```python
from build123d import *

# Parameters (mm, degrees)
BOSS_EXTRUDE1_DEPTH = 12.7
CUT_EXTRUDE1_START  = -13.7
SKETCH2_R           = 2.5
CUT_EXTRUDE1_DEPTH  = 14.7
LPATTERN1_COUNT     = 11
LPATTERN1_PITCH     = 38.608
CUT_EXTRUDE2_START  = -13.7
SKETCH3_R           = 2.5
CUT_EXTRUDE2_DEPTH  = 14.7
LPATTERN2_COUNT     = 11
LPATTERN2_PITCH     = 38.608
CUT_EXTRUDE3_START  = -13.7
SKETCH4_R           = 2.5
CUT_EXTRUDE3_DEPTH  = 14.7
LPATTERN3_COUNT     = 12
LPATTERN3_PITCH     = 38.608
CUT_EXTRUDE4_START  = -13.7
SKETCH5_R           = 2.5
CUT_EXTRUDE4_DEPTH  = 14.7
LPATTERN4_COUNT     = 12
LPATTERN4_PITCH     = 38.608


with BuildPart() as part:
    # Sketch1 → Boss-Extrude1 (new body)
    with BuildSketch(Plane(origin=(0, 0, 0), x_dir=(1, 0, 0), z_dir=(0, 1, 0))):
        Polygon((-199.53099264, 245.600086338), (200.46900736, 245.600086338), (200.46900736, 225.600086338), (240.46900736, 225.600086338), (240.46900736, -224.399913662), (200.46900736, -224.399913662), (200.46900736, -244.399913662), (-199.53099264, -244.399913662), (-199.53099264, -224.399913662), (-239.53099264, -224.399913662), (-239.53099264, 225.600086338), (-199.53099264, 225.600086338), align=None)
    extrude(amount=BOSS_EXTRUDE1_DEPTH)

    # Sketch2 → Cut-Extrude1 (cut)
    with BuildSketch(Plane(origin=(0, 12.7, 0), x_dir=(1, 0, 0), z_dir=(0, 1, 0)).offset(CUT_EXTRUDE1_START)):
        with Locations((-192.67299264, 235.440086338)):
            Circle(SKETCH2_R)
    cut_extrude1 = extrude(amount=CUT_EXTRUDE1_DEPTH, mode=Mode.SUBTRACT)

    # LPattern1: Cut-Extrude1 ×11
    with Locations(*[(i * LPATTERN1_PITCH, 0, 0) for i in range(1, LPATTERN1_COUNT)]):
        add(cut_extrude1, mode=Mode.SUBTRACT)

    # Sketch3 → Cut-Extrude2 (cut)
    with BuildSketch(Plane(origin=(0, 12.7, 0), x_dir=(1, 0, 0), z_dir=(0, 1, 0)).offset(CUT_EXTRUDE2_START)):
        with Locations((-192.67299264, -234.239913662)):
            Circle(SKETCH3_R)
    cut_extrude2 = extrude(amount=CUT_EXTRUDE2_DEPTH, mode=Mode.SUBTRACT)

    # LPattern2: Cut-Extrude2 ×11
    with Locations(*[(i * LPATTERN2_PITCH, 0, 0) for i in range(1, LPATTERN2_COUNT)]):
        add(cut_extrude2, mode=Mode.SUBTRACT)

    # Sketch4 → Cut-Extrude3 (cut)
    with BuildSketch(Plane(origin=(0, 12.7, 0), x_dir=(1, 0, 0), z_dir=(0, 1, 0)).offset(CUT_EXTRUDE3_START)):
        with Locations((230.30900736, 218.742086338)):
            Circle(SKETCH4_R)
    cut_extrude3 = extrude(amount=CUT_EXTRUDE3_DEPTH, mode=Mode.SUBTRACT)

    # LPattern3: Cut-Extrude3 ×12
    with Locations(*[(0, 0, i * LPATTERN3_PITCH) for i in range(1, LPATTERN3_COUNT)]):
        add(cut_extrude3, mode=Mode.SUBTRACT)

    # Sketch5 → Cut-Extrude4 (cut)
    with BuildSketch(Plane(origin=(0, 12.7, 0), x_dir=(1, 0, 0), z_dir=(0, 1, 0)).offset(CUT_EXTRUDE4_START)):
        with Locations((-229.37099264, 218.742086338)):
            Circle(SKETCH5_R)
    cut_extrude4 = extrude(amount=CUT_EXTRUDE4_DEPTH, mode=Mode.SUBTRACT)

    # LPattern4: Cut-Extrude4 ×12
    with Locations(*[(0, 0, i * LPATTERN4_PITCH) for i in range(1, LPATTERN4_COUNT)]):
        add(cut_extrude4, mode=Mode.SUBTRACT)


solid = part.part
```
Check sheet for the modelled part. Datum: model origin and axes. Units: mm. A direction names the side the tool comes from. Round coordinates to 2 decimals unless told otherwise and drop trailing zeros. Answer as CSV lines item,"result". Start each with the question number.
1) Scan line: probe 1 along Z at (x, y) = (205.5, 9.5). Record every from-to range of solid material in increasing order.
2) Draft check along Z on faces 6 (the face through (-219, 6, 224.4)), 7 (the face through (-2, 6, -245.6)), 8 (the face through (200.469, 6, -236)). Enter one of: +Z half, -Z half, draft (parallel to the pull), parting line (faces both ways), or undercut.
3) Tool access check on faces 1 (the face through (220, 6, -225.6)), 2 (the face through (200.469, 6, 234)), 3 (the face through (4, 12.7, -4)), 4 (the face through (-199.531, 6, -235)), 5 (the face through (-199.531, 6, 235)). Record the directions out of +Z, -Z, +X, -X, +Y, -Y that give a thin tool (end or side, any length) a straight path to the whole face; none if there is none.
4) Section check A-A (y = 7.5). Give the number of separate pieces and of enclosed holes in the cut face, then the cut area to 3 significant figures.
5) Depth check by flat-ended pin: pin 1 (4 mm diameter, centred on x = 38.98, z = -235.44, fed in from -Y). Enter the tip coordinate at first touch or a pass-through.
Determined:
1,probe 1,"-225.6 to 224.4"
2,face 6,"+Z half"
2,face 7,"-Z half"
2,face 8,"draft"
3,face 1,"-Z, +X, +Y, -Y"
3,face 2,"+Z, +X, +Y, -Y"
3,face 3,"+Z, -Z, +X, -X, +Y"
3,face 4,"-Z, -X, +Y, -Y"
3,face 5,"+Z, -X, +Y, -Y"
4,separate pieces,"1"
4,enclosed holes,"46"
4,area,"231,000 mm^2"
5,pin 1,"through"
